from build123d import *

# Parameters (mm, degrees)
SKETCH_1_R      = 8.15
SKETCH_1_R_2    = 2.15
EXTRUDE_1_DEPTH = 8.6
EXTRUDE_START   = 1
SKETCH_2_R      = 3.65
SKETCH_2_R_2    = 2.15
EXTRUDE_2_DEPTH = 1
CHAMFER_1_SIZE  = 1


with BuildPart() as part:
    # 草圖1 → 填料-伸長1 (new body)
    with BuildSketch(Plane.XY):
        with Locations(Location((0, 0, 0), (0, 0, 180))):
            Circle(SKETCH_1_R)
        with Locations(Location((0, 0, 0), (0, 0, 180))):
            Circle(SKETCH_1_R_2, mode=Mode.SUBTRACT)
    extrude(amount=EXTRUDE_1_DEPTH)

    # 草圖2 → 填料-伸長2 (add)
    with BuildSketch(Plane(origin=(0, 0, 0), x_dir=(-1, 0, 0), z_dir=(0, 0, -1)).offset(EXTRUDE_START)):
        with Locations(Location((0, 0, 0), (0, 0, 180))):
            Circle(SKETCH_2_R)
        Circle(SKETCH_2_R_2, mode=Mode.SUBTRACT)
    extrude(amount=-EXTRUDE_2_DEPTH)

    # 導角1
    chamfer_1_edges = [part.edges().sort_by_distance(p)[0] for p in [
        (-3.65, 0, 0),
    ]]
    chamfer(chamfer_1_edges, length=CHAMFER_1_SIZE - 0.0001)  # a hair under: the kernel refuses the full size


solid = part.part
The listing builds one solid part. Answer for the finished solid, in the listing's coordinates (mm). A direction names the side the tool comes from. Round coordinates to 2 decimals unless told otherwise and drop trailing zeros. Order: outer loops, then holes, each group sorted by start corner. A loop starts at its lowest first (then second) coordinate and runs counter-clockwise, first axis right, second up. Notation, with made-up numbers: M 31,28.25 L 76,28.25 A24 cw 76,47.25 Z; hole C 52,62 d3. An arc over 180 degrees is marked long. Answer in a Markdown table with one row per item. Add a question column.
1) Flat-ended cylindrical pins translate along their axes: pin 1 Ø1.5 at (x, y) = (-6.5, 4) entering from -Z; pin 2 Ø1.5 at (x, z) = (-2.5, 2.5) entering from -Y. Find the tip coordinate at first contact, or state that the pin passes through.
2) The part is cut by section C-C on z = 3.25. Determine the outline of the cut face in (x, y).
3) Consider line 1 along Y through (x, z) = (0, 2); line 2 along Z through (x, y) = (-1.25, -5); line 3 along Y through (x, z) = (0, -0.8). Determine where each line is inside the solid, lowest interval first. Write a range as from..to.
4) Which of the six approach directions +Z, -Z, +X, -X, +Y, -Y give full straight-line access (tool end or side, diameter ignored) to faces 1 (the face through (-2, 2, 8.6)), 2 (the face through (-4, 4, 0))?
5) The part is cut by section D-D on z = -0.5. Determine the outline of the cut face in (x, y), plus the area to 3 significant figures.
Findings below:
| question | item | result |
|---|---|---|
| 1 | pin 1 | stops at z = 0 |
| 1 | pin 2 | stops at y = -7.96 |
| 2 | outline | C 0,0 d16.3; hole C 0,0 d4.3 |
| 3 | line 1 | y = -8.15..-2.15, 2.15..8.15 |
| 3 | line 2 | z = 0..8.6 |
| 3 | line 3 | y = -3.85..-2.15, 2.15..3.85 |
| 4 | face 1 | +Z, +X, -X, +Y, -Y |
| 4 | face 2 | -Z |
| 5 | outline | C 0,0 d8.3; hole C 0,0 d4.3 |
| 5 | area | 39.6 mm² |
